Autodesk Inventor part; units mm, degrees
ref_plane "h1_XY" through (17.4625, 0, 17.526) normal (1, 0, 0) x (0, 0, -1)
ref_plane "h1_YZ" through (17.4625, 0, 17.526) normal (0, 0, -1) x (0, 1, 0)
ref_plane "h1_ZX" through (17.4625, 0, 17.526) normal (0, 1, 0) x (1, 0, 0)
sketch "Sketch_1" plane through (0, 0, 0) normal (1, 0, 0) x (0, 1, 0)
  line L0 (0, 17.526) -> (0, 3.0658)
  arc A0 (0, 3.0658) -> (3.0658, 0) centre (3.0658, 3.0658) ccw
  line L1 (3.0658, 0) -> (25.2679, 0)
  line L2 (25.2679, 0) -> (25.2679, 2.2784)
  line L3 (25.2679, 2.2784) -> (3.0658, 2.2784)
  arc A1 (2.2784, 3.0658) -> (3.0658, 2.2784) centre (3.0658, 3.0658) ccw
  line L4 (2.2784, 3.0658) -> (2.2784, 17.526)
  line L5 (2.2784, 17.526) -> (0, 17.526)
extrude "Extrusion1" add sketch "Sketch_1" along normal blind 34.925
sketch "Sketch_2" plane through (0, 0, 0) normal (0, 0, 1) x (1, 0, 0)
  line L0 (-6.985, -2.1057) -> (41.91, -2.1057)
  line L1 (41.91, -2.1057) -> (41.91, 33.6906)
  line L2 (41.91, 33.6906) -> (-6.985, 33.6906)
  line L3 (-6.985, 33.6906) -> (-6.985, -2.1057)
  line L4 (-2.2193, 0) -> (37.1443, 0)
  line L5 (37.1443, 0) -> (25.2694, 16.9886)
  arc A0 (25.2694, 16.9886) -> (9.6556, 16.9886) centre (17.4625, 11.5316) ccw
  line L6 (9.6556, 16.9886) -> (-2.2193, 0)
extrude "Extrusion2" cut sketch "Sketch_2" along normal blind 3.4176
sketch "Sketch3" plane through (34.925, 3.0658, 0) normal (0, 0, -1) x (-1, 0, 0)
  point P0 (17.4625, 11.2014)
hole "Drilling 1" at (17.4625, 14.2672, 0) direction (0, 0, 1) diameter 11.1887 depth 3.4176
sketch "Sketch_6" plane through (0, 0, 0) normal (0, 1, 0) x (-1, 0, 0)
  line L0 (17.4625, 14.351) -> (17.4625, 22.352)
  line L1 (17.4625, 22.352) -> (-3.175, 22.352)
  line L2 (-3.175, 22.352) -> (-3.175, 17.526)
  arc A0 (0, 14.351) -> (-3.175, 17.526) centre (-3.175, 14.351) ccw
  line L3 (0, 14.351) -> (17.4625, 14.351)
extrude "Extrusion3" cut sketch "Sketch_6" along normal blind 3.4176
sketch "Sketch_7" plane through (0, 0, 0) normal (0, 1, 0) x (-1, 0, 0)
  line L0 (-31.75, 22.352) -> (-52.3875, 22.352)
  line L1 (-52.3875, 22.352) -> (-52.3875, 14.351)
  line L2 (-52.3875, 14.351) -> (-34.925, 14.351)
  arc A0 (-31.75, 17.526) -> (-34.925, 14.351) centre (-31.75, 14.351) ccw
  line L3 (-31.75, 17.526) -> (-31.75, 22.352)
extrude "Extrusion4" cut sketch "Sketch_7" along normal blind 3.4176
sketch "Sketch_8" plane through (0, 0, 0) normal (0, 1, 0) x (-1, 0, 0)
  line L0 (3.4925, 12.0904) -> (-4.7625, 12.0904)
  arc A0 (-4.7625, 12.0904) -> (-4.7625, 7.2136) centre (-4.7625, 9.652) ccw
  line L1 (-4.7625, 7.2136) -> (3.4925, 7.2136)
  line L2 (3.4925, 7.2136) -> (3.4925, 12.0904)
extrude "Extrusion5" cut sketch "Sketch_8" along normal blind 3.4176
sketch "Sketch_9" plane through (0, 0, 0) normal (0, 1, 0) x (-1, 0, 0)
  arc A0 (-30.1625, 7.2136) -> (-30.1625, 12.0904) centre (-30.1625, 9.652) ccw
  line L0 (-30.1625, 12.0904) -> (-38.4175, 12.0904)
  line L1 (-38.4175, 12.0904) -> (-38.4175, 7.2136)
  line L2 (-38.4175, 7.2136) -> (-30.1625, 7.2136)
extrude "Extrusion6" cut sketch "Sketch_9" along normal blind 3.4176
sketch "Sketch_10" plane through (11.1125, 0, 0) normal (1, 0, 0) x (0, 0, -1)
  arc A0 (-4.5568, 1.8456) -> (-1.8456, 4.5568) centre (-3.0658, 3.0658) ccw
  line L0 (-1.8456, 4.5568) -> (-2.2784, 4.5568)
  line L1 (-2.2784, 4.5568) -> (-4.5568, 2.2784)
  line L2 (-4.5568, 2.2784) -> (-4.5568, 1.8456)
extrude "Extrusion7" add sketch "Sketch_10" along normal blind 2.2784
sketch "Sketch_14" plane through (23.8125, 0, 0) normal (1, 0, 0) x (0, 0, -1)
  arc A0 (-4.5568, 1.8456) -> (-1.8456, 4.5568) centre (-3.0658, 3.0658) ccw
  line L0 (-1.8456, 4.5568) -> (-2.2784, 4.5568)
  line L1 (-2.2784, 4.5568) -> (-4.5568, 2.2784)
  line L2 (-4.5568, 2.2784) -> (-4.5568, 1.8456)
extrude "Extrusion8" add sketch "Sketch_14" against normal blind 2.2784
ref_plane "h1_XY" through (17.4625, 0, 17.526) normal (1, 0, 0) x (0, 0, -1)
ref_plane "h1_YZ" through (17.4625, 0, 17.526) normal (0, 0, -1) x (0, 1, 0)
ref_plane "h1_ZX" through (17.4625, 0, 17.526) normal (0, 1, 0) x (1, 0, 0)
ref_plane "d1_XY" through (17.4625, 8.6728, 0) normal (1, 0, 0) x (0, 0, -1)
ref_plane "d1_YZ" through (17.4625, 8.6728, 0) normal (0, 0, -1) x (0, 1, 0)
ref_plane "d1_ZX" through (17.4625, 8.6728, 0) normal (0, 1, 0) x (1, 0, 0)
ref_plane "h2_XY" through (17.4625, 2.2784, 17.526) normal (1, 0, 0) x (0, 0, -1)
ref_plane "h2_YZ" through (17.4625, 2.2784, 17.526) normal (0, 0, -1) x (0, 1, 0)
ref_plane "h2_ZX" through (17.4625, 2.2784, 17.526) normal (0, 1, 0) x (1, 0, 0)
ref_plane "d2_XY" through (17.4625, 19.8615, 0) normal (1, 0, 0) x (0, 0, -1)
ref_plane "d2_YZ" through (17.4625, 19.8615, 0) normal (0, 0, -1) x (0, 1, 0)
ref_plane "d2_ZX" through (17.4625, 19.8615, 0) normal (0, 1, 0) x (1, 0, 0)
ref_plane "h3_XY" through (17.4625, 14.2672, 2.2784) normal (1, 0, 0) x (0, 0, -1)
ref_plane "h3_YZ" through (17.4625, 14.2672, 2.2784) normal (0, 0, -1) x (0, 1, 0)
ref_plane "h3_ZX" through (17.4625, 14.2672, 2.2784) normal (0, 1, 0) x (1, 0, 0)
ref_plane "h4_XY" through (17.4625, 21.0566, 2.2784) normal (1, 0, 0) x (0, 0, -1)
ref_plane "h4_YZ" through (17.4625, 21.0566, 2.2784) normal (0, 0, -1) x (0, 1, 0)
ref_plane "h4_ZX" through (17.4625, 21.0566, 2.2784) normal (0, 1, 0) x (1, 0, 0)
ref_plane "h5_XY" through (34.925, 3.175, 0) normal (1, 0, 0) x (0, 0, -1)
ref_plane "h5_YZ" through (34.925, 3.175, 0) normal (0, 0, -1) x (0, 1, 0)
ref_plane "h5_ZX" through (34.925, 3.175, 0) normal (0, 1, 0) x (1, 0, 0)
ref_plane "h6_XY" through (34.925, 0, 0) normal (1, 0, 0) x (0, 0, -1)
ref_plane "h6_YZ" through (34.925, 0, 0) normal (0, 0, -1) x (0, 1, 0)
ref_plane "h6_ZX" through (34.925, 0, 0) normal (0, 1, 0) x (1, 0, 0)
ref_plane "l1_XY" through (0, 0, 0) normal (0, 1, 0) x (1, 0, 0)
ref_plane "l1_YZ" through (0, 0, 0) normal (1, 0, 0) x (0, 0, -1)
ref_plane "l1_ZX" through (0, 0, 0) normal (0, 0, -1) x (0, 1, 0)
ref_plane "l2_XY" through (34.925, 0, 0) normal (0, 1, 0) x (1, 0, 0)
ref_plane "l2_YZ" through (34.925, 0, 0) normal (1, 0, 0) x (0, 0, -1)
ref_plane "l2_ZX" through (34.925, 0, 0) normal (0, 0, -1) x (0, 1, 0)
ref_plane "l3_XY" through (0, 0, 17.526) normal (0, 1, 0) x (1, 0, 0)
ref_plane "l3_YZ" through (0, 0, 17.526) normal (1, 0, 0) x (0, 0, -1)
ref_plane "l3_ZX" through (0, 0, 17.526) normal (0, 0, -1) x (0, 1, 0)
ref_plane "l4_XY" through (0, 0, 9.652) normal (0, 1, 0) x (1, 0, 0)
ref_plane "l4_YZ" through (0, 0, 9.652) normal (1, 0, 0) x (0, 0, -1)
ref_plane "l4_ZX" through (0, 0, 9.652) normal (0, 0, -1) x (0, 1, 0)
ref_plane "l5_XY" through (4.7625, 0, 9.652) normal (0, 1, 0) x (1, 0, 0)
ref_plane "l5_YZ" through (4.7625, 0, 9.652) normal (1, 0, 0) x (0, 0, -1)
ref_plane "l5_ZX" through (4.7625, 0, 9.652) normal (0, 0, -1) x (0, 1, 0)
ref_plane "l6_XY" through (30.1625, 0, 9.652) normal (0, 1, 0) x (1, 0, 0)
ref_plane "l6_YZ" through (30.1625, 0, 9.652) normal (1, 0, 0) x (0, 0, -1)
ref_plane "l6_ZX" through (30.1625, 0, 9.652) normal (0, 0, -1) x (0, 1, 0)
ref_plane "l7_XY" through (30.1625, 0, 12.0904) normal (0, 1, 0) x (1, 0, 0)
ref_plane "l7_YZ" through (30.1625, 0, 12.0904) normal (1, 0, 0) x (0, 0, -1)
ref_plane "l7_ZX" through (30.1625, 0, 12.0904) normal (0, 0, -1) x (0, 1, 0)
ref_plane "l8_XY" through (30.1625, 0, 7.2136) normal (0, 1, 0) x (1, 0, 0)
ref_plane "l8_YZ" through (30.1625, 0, 7.2136) normal (1, 0, 0) x (0, 0, -1)
ref_plane "l8_ZX" through (30.1625, 0, 7.2136) normal (0, 0, -1) x (0, 1, 0)
ref_plane "mounting_bracket_XY" through (17.4625, 14.2672, 2.2784) normal (0, 0, 1) x (1, 0, 0)
ref_plane "mounting_bracket_YZ" through (17.4625, 14.2672, 2.2784) normal (1, 0, 0) x (0, 1, 0)
ref_plane "mounting_bracket_ZX" through (17.4625, 14.2672, 2.2784) normal (0, 1, 0) x (0, 0, 1)
ref_plane "mounting_bracket_1_XY" through (17.4625, 14.2672, 0) normal (0, 0, 1) x (1, 0, 0)
ref_plane "mounting_bracket_1_YZ" through (17.4625, 14.2672, 0) normal (1, 0, 0) x (0, 1, 0)
ref_plane "mounting_bracket_1_ZX" through (17.4625, 14.2672, 0) normal (0, 1, 0) x (0, 0, 1)
properties part number "D-770"
Input: part model. Units: mm. Frame: model coordinates. A direction names the side the tool comes from. Give positions to 0.01 mm unless a question says otherwise; leave off trailing zeros. Loops run counter-clockwise (first coordinate to the right, second up) from the corner with the lowest first, then second, coordinate; pieces in that order, holes last. Notation, with made-up numbers: M 51,63 L 68,63 A29 ccw 68,83 Z; hole C 42,71 d4. An arc over 180 degrees is marked long. Answer as CSV lines item,"result". Start each with the question number.
1. Section C-C on z = 1.5. Return loops of the section in (x, y) (1 decimal).
2. Pull-direction query (X, two-part tool) for faces 1 (the face through (0, 1, 13)), 2 (the face through (17, 8, 0)), 3 (the face through (34.02, 1.12, 16.57)), 4 (the face through (21.534, 3, 3)); classes: released by +X, released by -X, zero draft, split by the parting line, or undercut.
3. Line query: L1, parallel to Z at x = 26, y = 10.25; L2, parallel to Y at x = 12, z = 3.25. Output: solid intervals per line, ascending.
4. Pin query (flat end, axial travel): P1, Ø5, axis at y = 3.5, z = 6, coming from the +X side (3 decimals); P2, Ø1.8, axis at x = 2, y = 1, coming from the -Z side; P3, Ø4, axis at y = 9.5, z = 3.5, coming from the -X side; P4, Ø0.7, axis at x = 33.5, y = 0.5, coming from the +Z side. Return the tip coordinate at first contact, or that it passes through.
5. Section B-B on x = 5.5. Return loops of the section in (y, z), plus the area to 3 significant figures.
6. Section A-A on y = 13. Return loops of the section in (x, z).
7. Section D-D on x = 18.5. Return loops of the section in (y, z), plus the area to 3 significant figures.
8. Reachability of faces 5 (the face through (12.236, 3.434, 3.402)), 6 (the face through (17, 8, 2.278)), 7 (the face through (11.112, 3, 3)), 8 (the face through (33, 1, 12.09)), 9 (the face through (2, 1, 7.214)) from +Z, -Z, +X, -X, +Y, -Y: full face, straight path, thin tool, end or side. Return the list, or none.
Computed values:
1,outline,"M 0,0.4 L 34.9,0.4 L 34.9,3.2 L 25.3,17 A9.5 ccw 9.7,17 L 0,3.2 Z; hole C 17.5,14.3 d11.2"
2,face 1,"released by -X"
2,face 2,"zero draft"
2,face 3,"released by +X"
2,face 4,"undercut"
3,L1,"z = 0 to 2.28"
3,L2,"y = 0 to 3.59"
4,P1,"stops at x = 34.925"
4,P2,"stops at z = 0.23"
4,P3,"stops at x = 3.31"
4,P4,"stops at z = 17.2"
5,outline,"M 0,3.07 A3.07 ccw 3.07,0 L 11.04,0 L 11.04,2.28 L 3.07,2.28 A0.79 cw 2.28,3.07 L 2.28,7.33 L 0,7.33 Z; M 0,11.98 L 2.28,11.98 L 2.28,17.53 L 0,17.53 Z"
5,area,"47.4 mm²"
6,outline,"M 6.87,0 L 12.01,0 L 12.01,2.28 L 6.87,2.28 Z; M 22.91,0 L 28.06,0 L 28.06,2.28 L 22.91,2.28 Z"
7,outline,"M 0,3.07 A3.07 ccw 3.07,0 L 8.77,0 L 8.77,2.28 L 3.07,2.28 A0.79 cw 2.28,3.07 L 2.28,17.53 L 0,17.53 Z; M 19.76,0 L 21,0 L 21,2.28 L 19.76,2.28 Z"
7,area,"55.7 mm²"
8,face 5,"+Z, +X, -X, +Y"
8,face 6,"+Z, +Y"
8,face 7,"+Z, -X, +Y"
8,face 8,"+X, +Y, -Y"
8,face 9,"-X, +Y, -Y"
